Here's how the part is built. I have some questions about the finished solid (model axes, mm). Coordinates: 2 decimals unless noted, no trailing zeros. Loops run counter-clockwise (first coordinate to the right, second up) from the corner with the lowest first, then second, coordinate; pieces in that order, holes last. Notation, with made-up numbers: M 73.5,34.25 L 99.5,34.25 A12 ccw 99.5,49.25 Z; hole C -30,52 d1. An arc over 180 degrees is marked long. Use one line per item in the form item = value. Start each with the question number.
(1) Please list where these lines run through material, in increasing order: L1, parallel to X at y = -260.5, z = -5.75; L2, parallel to Y at x = 227, z = -15.75; L3, parallel to Y at x = 126, z = -13.75.
(2) Imagine slicing it at C-C, the plane z = -4. Please give me the cut outline in (x, y), and give its area (3 significant figures).
(3) Imagine slicing it at A-A, the plane x = -381. Please give me the cut outline in (y, z).
(4) Will these pins go through, and if not, where does the flat tip stop? P1, Ø1.5, axis at y = 195, z = -4, coming from the +X side; P2, Ø1, axis at y = 107.5, z = -16, coming from the +X side; P3, Ø5, axis at x = 33.5, z = -9.5, coming from the +Y side.
Autodesk Inventor part; units mm, degrees
ref_plane "YZ Plane" through (0, 0, 0) normal (1, 0, 0) x (0, 1, 0)
ref_plane "XZ Plane" through (0, 0, 0) normal (0, 1, 0) x (-1, 0, 0)
ref_plane "XY Plane" through (0, 0, 0) normal (0, 0, 1) x (1, 0, 0)
sketch "Sketch1" plane through (0, 0, 0) normal (0, 0, 1) x (1, 0, 0)
  line L0 (457.2, -457.2) -> (-457.2, -457.2)
  line L1 (-457.2, -457.2) -> (-457.2, 457.2)
  line L2 (-457.2, 457.2) -> (457.2, 457.2)
  line L3 (457.2, 457.2) -> (457.2, -457.2)
  point P0 (0, 0)
  dimension "d0" = 914.4
  dimension "d1" = 914.4
  dimension "d2" = 457.2
  dimension "d3" = 457.2
extrude "Extrusion1" add sketch "Sketch1" against normal blind 19.05 draft -55
extrude "Extrusion2" add sketch "Sketch1" along normal blind 6.35
equation "\"d1\" = d0"
properties part number "TableTop" material "Wood (Walnut)"
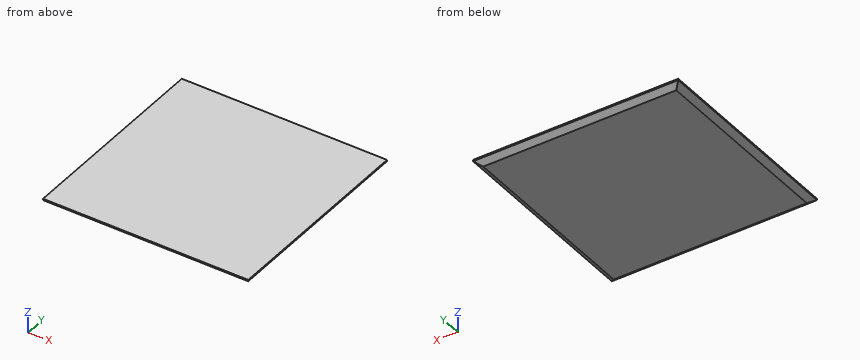
Answer:
q1.L1 = -448.99 to 448.99
q1.L2 = -434.71 to 434.71
q1.L3 = -437.56 to 437.56
q2.outline = M -451.49,-451.49 L 451.49,-451.49 L 451.49,451.49 L -451.49,451.49 Z
q2.area = 815,000 mm²
q3.outline = M -457.2,0 L -429.99,-19.05 L 429.99,-19.05 L 457.2,0 L 457.2,6.35 L -457.2,6.35 Z
q4.P1 = 452.56
q4.P2 = 435.06
q4.P3 = 447.2
